Input: dimensioned drawing with shaded views. Units: mm. Origin: part minimum x, y, z. Give positions to 0.01 mm unless a question says otherwise; leave off trailing zeros. Write each loop counter-clockwise with the first axis right and the second up, starting at its lowest first coordinate (ties: lowest second). Pieces come first, ordered by that corner, then holes.
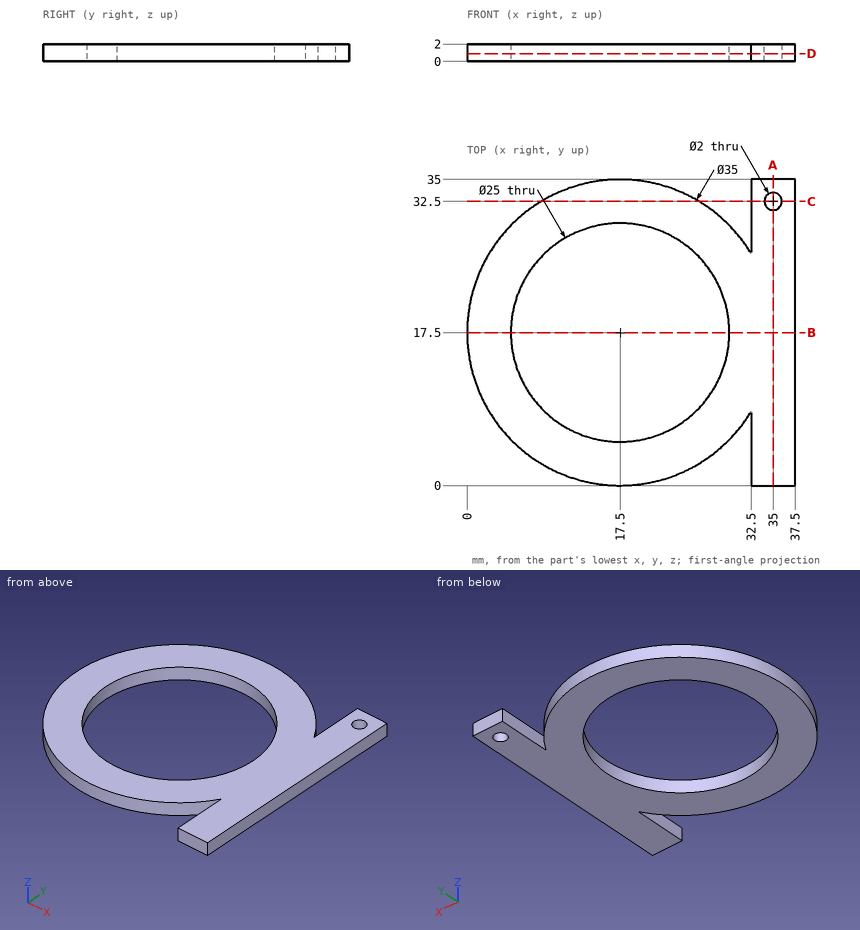
Item 1: Section D-D (z = 0.9). Return loops of the section in (x, y).
Item 2: Pin query (flat end, axial travel): pin 1 (1 mm diameter, centred on y = 29.5, z = 1.5, fed in from -X); pin 2 (0.6 mm diameter, centred on y = 6, z = 1, fed in from -X); pin 3 (1.6 mm diameter, centred on x = 35, y = 32.5, fed in from -Z). Return the tip coordinate at first contact, or that it passes through.
Item 3: Section A-A (x = 35). Return loops of the section in (y, z), and give its area (3 significant figures).
Item 4: Ray query, line 1 (Y direction, x = 17.5, z = 1.2); line 2 (X direction, y = 32, z = 1.5); line 3 (Y direction, x = 35, z = 1.55). Return the intervals inside material, ascending.
Item 5: Section B-B (y = 17.5). Return loops of the section in (x, z).
Item 6: Section C-C (y = 32.5). Return loops of the section in (x, z).
Solved:
1. outline: (32.5, 0) - (37.5, 0) - (37.5, 35) - (32.5, 35) - (32.5, 26.51) arc R17.5 ccw (long way) to (32.5, 8.49) - close; hole circle Ø25 at (17.5, 17.5); hole circle Ø2 at (35, 32.5)
2. pin 1: stops at x = 4.31
2. pin 2: stops at x = 4.05
2. pin 3: passes through
3. outline: (0, 0) - (31.5, 0) - (31.5, 2) - (0, 2) - close; (33.5, 0) - (35, 0) - (35, 2) - (33.5, 2) - close
3. area: 66.0 mm2
4. line 1: y = 0 to 5, 30 to 35
4. line 2: x = 7.7 to 27.3, 32.5 to 34.13, 35.87 to 37.5
4. line 3: y = 0 to 31.5, 33.5 to 35
5. outline: (0, 0) - (5, 0) - (5, 2) - (0, 2) - close; (30, 0) - (37.5, 0) - (37.5, 2) - (30, 2) - close
6. outline: (8.49, 0) - (26.51, 0) - (26.51, 2) - (8.49, 2) - close; (32.5, 0) - (34, 0) - (34, 2) - (32.5, 2) - close; (36, 0) - (37.5, 0) - (37.5, 2) - (36, 2) - close
